Source: CAD feature listing. Evaluate the final solid. Frame: model axes, mm. A direction names the side the tool comes from. Coordinates: 2 decimals unless noted, no trailing zeros. Loops run counter-clockwise (first coordinate to the right, second up) from the corner with the lowest first, then second, coordinate; pieces in that order, holes last.
```python
from build123d import *

# Parameters (mm, degrees)
PAD014_DEPTH    = 11.43
SKETCH067_W     = 1.905
SKETCH067_H     = 17.145
PAD015_DEPTH    = 1.27
PAD016_DEPTH    = 5.08
SKETCH074_R     = 3.175
SKETCH074_R_2   = 2.2225
SKETCH074_W     = 2.54
SKETCH074_H     = 4.445
POCKET012_DEPTH = 5.08


with BuildPart() as part:
    # Sketch066 → Pad014 (new body)
    with BuildSketch(Plane.XZ):
        with BuildLine():
            ThreePointArc((-6.985, 14.9225), (-11.475128, 13.062628), (-13.335, 8.5725))
            Line((-13.335, -8.5725), (-13.335, 8.5725))
            ThreePointArc((-13.335, -8.5725), (-11.475128, -13.062628), (-6.985, -14.9225))
            Line((6.985, -14.9225), (-6.985, -14.9225))
            ThreePointArc((6.985, -14.9225), (11.475128, -13.062628), (13.335, -8.5725))
            Line((13.335, 8.5725), (13.335, -8.5725))
            ThreePointArc((13.335, 8.5725), (11.475128, 13.062628), (6.985, 14.9225))
            Line((-6.985, 14.9225), (6.985, 14.9225))
        make_face()
    extrude(amount=-PAD014_DEPTH)

    # Sketch067 (on Face10 of Pad014) → Pad015 (join)
    with BuildSketch(Plane(origin=(0, 11.43, 0), x_dir=(1, 0, 0), z_dir=(0, 1, 0))):
        with Locations((-12.3825, 0)):
            Rectangle(SKETCH067_W, SKETCH067_H)
        with Locations((12.3825, 0)):
            Rectangle(SKETCH067_W, SKETCH067_H)
    extrude(amount=PAD015_DEPTH)

    # Sketch068 (on Face5 of Pad015) → Pad016 (join)
    with BuildSketch(Plane(origin=(0, 11.43, 0), x_dir=(1, 0, 0), z_dir=(0, 1, 0))):
        with BuildLine():
            ThreePointArc((-0.3175, 7.9375), (-1.215526, 7.565526), (-1.5875, 6.6675))
            Line((-1.5875, -6.6675), (-1.5875, 6.6675))
            ThreePointArc((-1.5875, -6.6675), (-1.215526, -7.565526), (-0.3175, -7.9375))
            Line((0.3175, -7.9375), (-0.3175, -7.9375))
            ThreePointArc((0.3175, -7.9375), (1.215526, -7.565526), (1.5875, -6.6675))
            Line((1.5875, 6.6675), (1.5875, -6.6675))
            ThreePointArc((1.5875, 6.6675), (1.215526, 7.565526), (0.3175, 7.9375))
            Line((-0.3175, 7.9375), (0.3175, 7.9375))
        make_face()
    extrude(amount=PAD016_DEPTH)

    # Sketch074 (on Face5 of Pad016) → Pocket012 (cut)
    with BuildSketch(Plane(origin=(0, 11.43, 0), x_dir=(1, 0, 0), z_dir=(0, 1, 0))):
        with Locations((-6.731, -8.89)):
            Circle(SKETCH074_R)
        with Locations((6.731, 8.89)):
            Circle(SKETCH074_R)
        with Locations((-6.35, 0)):
            Circle(SKETCH074_R_2)
        with Locations((6.35, 0)):
            Circle(SKETCH074_R_2)
        with Locations((0, -10.922)):
            Rectangle(SKETCH074_W, SKETCH074_H)
        with Locations((0, 10.922)):
            Rectangle(SKETCH074_W, SKETCH074_H)
    extrude(amount=-POCKET012_DEPTH, mode=Mode.SUBTRACT)


with BuildPart() as part_1:
    # Body011 placement: moved
    add(part.part.moved(Location((17.78, 159.385, 0))))


solid = part_1.part
```
Q1. Section query A-A on y = 173. Return the cut outline in (x, z), then the cut area to 3 significant figures.
Q2. Section query C-C on x = 26. Return the cut outline in (y, z) (3 decimals).
Q3. Section query D-D on z = -9.25. Return the cut outline in (x, y) (3 decimals).
Q4. First-contact query: pin 1 Ø0.6 at (x, y) = (29.5, 171.5) entering from -Z; pin 2 Ø1 at (x, z) = (6, 4) entering from +Y (3 decimals); pin 3 Ø2 at (x, z) = (18, 11) entering from +Y (3 decimals). Flat tips, straight axial feed; report the tip coordinate or a pass-through.
Q5. Draft query along Z for faces 4 (the cylindrical face through (29.21, 165.02, -13.11)), 5 (the flat face through (19.05, 168, 11)), 6 (the flat face through (18, 175.895, 0)), 7 (the flat face through (30, 171, 8.572)). Return one class per face: released by +Z, released by -Z, zero draft, split by the parting line, or undercut.
Q6. Material intervals for line 1 along X through (y, z) = (167.3, 8.89); line 2 along X through (y, z) = (167.55, 0) (1 decimal); line 3 along Z through (x, y) = (18.75, 166.5), sorted ascending.
Q7. Reachability of faces 1 (the flat face through (5, 171, 8.572)), 2 (the flat face through (16.51, 168, -11)), 3 (the cylindrical face through (18.986, 173.319, 7.575)) from +Z, -Z, +X, -X, +Y, -Y: full face, straight path, thin tool, end or side. Return the list, or none.
Resolved:
1. outline: (16.19, -6.67) arc R1.27 ccw to (17.46, -7.94) - (18.1, -7.94) arc R1.27 ccw to (19.37, -6.67) - (19.37, 6.67) arc R1.27 ccw to (18.1, 7.94) - (17.46, 7.94) arc R1.27 ccw to (16.19, 6.67) - close
1. area: 49.0 mm2
2. outline: (159.385, -14.801) - (170.815, -14.801) - (170.815, -11.694) - (165.735, -11.694) - (165.735, -6.086) - (170.815, -6.086) - (170.815, -1.201) - (165.735, -1.201) - (165.735, 1.201) - (170.815, 1.201) - (170.815, 14.801) - (159.385, 14.801) - close
3. outline: (4.481, 159.385) - (31.079, 159.385) - (31.079, 170.815) - (27.666, 170.815) - (27.666, 165.735) - (21.356, 165.735) - (21.356, 170.815) - (19.05, 170.815) - (19.05, 165.735) - (16.51, 165.735) - (16.51, 170.815) - (4.481, 170.815) - close
4. pin 1: stops at z = -8.57
4. pin 2: stops at y = 172.085
4. pin 3: stops at y = 165.735
5. face 4: released by -Z
5. face 5: undercut
5. face 6: zero draft
5. face 7: released by +Z
6. line 1: x = 4.45 to 7.87, 14.22 to 16.51, 19.05 to 31.11
6. line 2: x = 4.4 to 9.2, 13.7 to 21.9, 26.4 to 31.1
6. line 3: z = -14.92 to -13.14, -8.7 to 8.7, 13.14 to 14.92
7. face 1: +Z, +X, -X, +Y
7. face 2: +Y
7. face 3: +Z, +Y
